from build123d import *

# Parameters (mm, degrees)
SKETCH_1_W          = 53
SKETCH_1_H          = 50
EXTRUDE_1_DEPTH     = 3
CUT_EXTRUDE_1_DEPTH = 4
SKETCH_3_W          = 3
SKETCH_3_H          = 50
EXTRUDE_2_DEPTH     = 83
CUT_EXTRUDE_2_DEPTH = 54
EXTRUDE_3_DEPTH     = 2
EXTRUDE_4_DEPTH     = 2
FILLET_1_R          = 5


with BuildPart() as part:
    # 草图1 → 凸台-拉伸1 (new body)
    with BuildSketch(Plane(origin=(0, 0, 0), x_dir=(1, 0, 0), z_dir=(0, 1, 0))):
        Rectangle(SKETCH_1_W, SKETCH_1_H)
    extrude(amount=EXTRUDE_1_DEPTH)

    # 草图2 → 切除-拉伸1 (cut, through all)
    with BuildSketch(Plane(origin=(0, 3, 0), x_dir=(1, 0, 0), z_dir=(0, 1, 0))):
        with BuildLine():
            Line((-17.5, 21.514185104), (17.5, 21.514185104))
            ThreePointArc((17.5, 21.514185104), (20, 19.014185104), (17.5, 16.514185104))
            Line((17.5, 16.514185104), (-17.5, 16.514185104))
            ThreePointArc((-17.5, 16.514185104), (-20, 19.014185104), (-17.5, 21.514185104))
        make_face()
        with BuildLine():
            Line((-17.5, -21.514185104), (17.5, -21.514185104))
            ThreePointArc((17.5, -21.514185104), (20, -19.014185104), (17.5, -16.514185104))
            Line((17.5, -16.514185104), (-17.5, -16.514185104))
            ThreePointArc((-17.5, -16.514185104), (-20, -19.014185104), (-17.5, -21.514185104))
        make_face()
    extrude(amount=-CUT_EXTRUDE_1_DEPTH, mode=Mode.SUBTRACT)

    # 草图3 → 凸台-拉伸2 (add)
    with BuildSketch(Plane(origin=(0, 3, 0), x_dir=(1, 0, 0), z_dir=(0, 1, 0))):
        with Locations((-25, 0)):
            Rectangle(SKETCH_3_W, SKETCH_3_H)
    extrude(amount=EXTRUDE_2_DEPTH)

    # 草图4 → 切除-拉伸2 (cut, through all)
    with BuildSketch(Plane.ZY.offset(26.5)):
        with BuildLine():
            Line((-13.921207139, 82), (-13.921207139, 34))
            ThreePointArc((-13.921207139, 34), (-15.521207139, 32.4), (-17.121207139, 34))
            Line((-17.121207139, 34), (-17.121207139, 82))
            ThreePointArc((-17.121207139, 82), (-15.521207139, 83.6), (-13.921207139, 82))
        make_face()
        with BuildLine():
            Line((11.1, 65.5), (11.1, 50.5))
            ThreePointArc((11.1, 50.5), (0, 39.4), (-11.1, 50.5))
            Line((-11.1, 50.5), (-11.1, 65.5))
            ThreePointArc((-11.1, 65.5), (0, 76.6), (11.1, 65.5))
        make_face()
        with BuildLine():
            Line((17.078792861, 82), (17.078792861, 34))
            ThreePointArc((17.078792861, 34), (15.478792861, 32.4), (13.878792861, 34))
            Line((13.878792861, 34), (13.878792861, 82))
            ThreePointArc((13.878792861, 82), (15.478792861, 83.6), (17.078792861, 82))
        make_face()
    extrude(amount=-CUT_EXTRUDE_2_DEPTH, mode=Mode.SUBTRACT)

    # 草图5 → 凸台-拉伸3 (add)
    with BuildSketch(Plane.XY.offset(25)):
        Polygon((-23.5, 18), (-8.5, 3), (-23.5, 3), align=None)
    extrude(amount=-EXTRUDE_3_DEPTH)

    # 草图7 → 凸台-拉伸4 (add)
    with BuildSketch(Plane(origin=(0, 0, -25), x_dir=(-1, 0, 0), z_dir=(0, 0, -1))):
        Polygon((23.5, 18), (8.5, 3), (23.5, 3), align=None)
    extrude(amount=-EXTRUDE_4_DEPTH)

    # 圆角1
    fillet_1_edges = [part.edges().sort_by_distance(p)[0] for p in [
        (-25, 86, 25),
        (-25, 86, -25),
        (26.5, 1.5, 25),
        (26.5, 1.5, -25),
    ]]
    fillet(fillet_1_edges, radius=FILLET_1_R)


solid = part.part
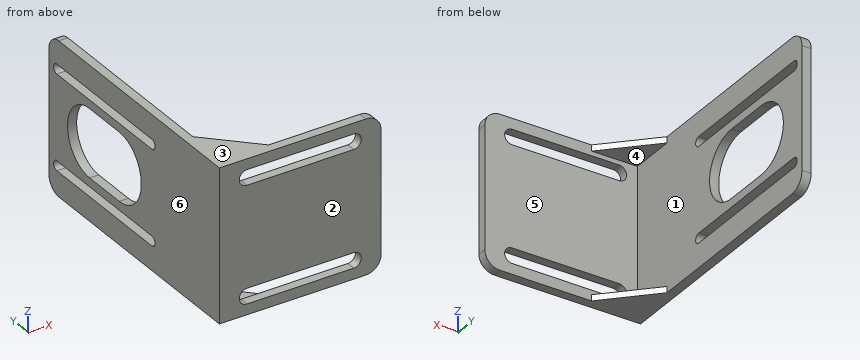
Can you work these out from the model? Positions are in its coordinate system, mm. Face numbers are marked on the shaded views. A direction names the side the tool comes from. Coordinates: 2 decimals unless noted, no trailing zeros. Order: outer loops, then holes, each group sorted by start corner. A loop starts at its lowest first (then second) coordinate and runs counter-clockwise, first axis right, second up. Notation, with made-up numbers: (29, 79) - (37, 79) arc R17 ccw to (37, 108) - close; hole circle Ø2 at (20, 45). An arc over 180 degrees is marked (long way). Answer as a JSON object with one key per item and string values. Group by question number.
Q1. Will these pins go through, and if not, where does the flat tip stop? P1, Ø2, axis at y = 43, z = 7, coming from the +X side; P2, Ø12, axis at x = -12.5, y = 13, coming from the +Z side; P3, Ø25, axis at x = -9, z = -4, coming from the +Y side.
Q2. I need wall thicknesses on line 1 (Z direction, x = -23, y = 17); line 2 (X direction, y = 81.5, z = -7.5); line 3 (Y direction, x = 20.5, z = 1). Which ranges of each line are inside material? Lowest first, please. Write a range as from..to.
Q3. We'd pull the mould along Z, two halves only. Please class the marked faces 1, 2, 3 and 4: +Z half, -Z half, draft (parallel to the pull), parting line (faces both ways), or undercut.
Q4. On a 3-axis mill with a long thin cutter (end or side, diameter ignored), from which of +Z, -Z, +X, -X, +Y, -Y can I reach the whole of each face in a straight line? I mean the marked faces 5 and 6. Say none if no direction works.
Q5. Imagine slicing it at D-D (y = 35). Please give me the cut outline in (x, z), and give its area (3 significant figures).
Q6. Imagine slicing it at C-C (z = 0). Please give me the cut outline in (x, y).
Q7. Imagine slicing it at B-B (y = 64). Please give me the cut outline in (x, z).
Q8. Imagine slicing it at A-A (x = 10.5). Please give me the cut outline in (y, z).
Determined:
{
 "1": {"P1": "stops at x = -23.5", "P2": "stops at z = 25", "P3": "stops at y = 3"},
 "2": {"line 1": "z = -25..-23, 23..25", "line 2": "x = -26.5..-23.5", "line 3": "y = 0..3"},
 "3": {"face 1": "undercut", "face 2": "draft", "face 3": "+Z half", "face 4": "undercut"},
 "4": {"face 5": "+X, +Y", "face 6": "+Z, -Z, -X, +Y, -Y"},
 "5": {"outline": "(-26.5, -25) - (-23.5, -25) - (-23.5, -17.12) - (-26.5, -17.12) - close; (-26.5, -13.92) - (-23.5, -13.92) - (-23.5, 13.88) - (-26.5, 13.88) - close; (-26.5, 17.08) - (-23.5, 17.08) - (-23.5, 25) - (-26.5, 25) - close", "area": "131 mm2"},
 "6": {"outline": "(-26.5, 0) - (26.5, 0) - (26.5, 3) - (-23.5, 3) - (-23.5, 39.4) - (-26.5, 39.4) - close; (-26.5, 76.6) - (-23.5, 76.6) - (-23.5, 86) - (-26.5, 86) - close"},
 "7": {"outline": "(-26.5, -25) - (-23.5, -25) - (-23.5, -17.12) - (-26.5, -17.12) - close; (-26.5, -13.92) - (-23.5, -13.92) - (-23.5, -11.1) - (-26.5, -11.1) - close; (-26.5, 11.1) - (-23.5, 11.1) - (-23.5, 13.88) - (-26.5, 13.88) - close; (-26.5, 17.08) - (-23.5, 17.08) - (-23.5, 25) - (-26.5, 25) - close"},
 "8": {"outline": "(0, -25) - (3, -25) - (3, -21.51) - (0, -21.51) - close; (0, -16.51) - (3, -16.51) - (3, 16.51) - (0, 16.51) - close; (0, 21.51) - (3, 21.51) - (3, 25) - (0, 25) - close"}
}
